```python
from build123d import *

# Parameters (mm, degrees)
SKETCH1_R           = 12.25
BOSS_EXTRUDE1_DEPTH = 280
CUT_EXTRUDE1_DEPTH  = 20


with BuildPart() as part:
    # Sketch1 → Boss-Extrude1 (new body)
    with BuildSketch(Plane.XY):
        Circle(SKETCH1_R)
    extrude(amount=BOSS_EXTRUDE1_DEPTH)

    # Sketch2 → Cut-Extrude1 (cut)
    with BuildSketch(Plane.XY.offset(280)):
        with BuildLine():
            Line((1, 6.75), (-1, 6.75))
            Line((-1, 6.75), (-1, 8.692669325))
            ThreePointArc((-1, 8.692669325), (-3.348480033, 8.083945909), (-5.439538645, 6.853752208))
            Line((-5.439538645, 6.853752208), (-4.065863992, 5.480077554))
            Line((-4.065863992, 5.480077554), (-5.480077554, 4.065863992))
            Line((-5.480077554, 4.065863992), (-6.853752208, 5.439538645))
            ThreePointArc((-6.853752208, 5.439538645), (-8.083945909, 3.348480033), (-8.692669325, 1))
            Line((-8.692669325, 1), (-6.75, 1))
            Line((-6.75, 1), (-6.75, -1))
            Line((-6.75, -1), (-8.692669325, -1))
            ThreePointArc((-8.692669325, -1), (-8.083945909, -3.348480033), (-6.853752208, -5.439538645))
            Line((-6.853752208, -5.439538645), (-5.480077554, -4.065863992))
            Line((-5.480077554, -4.065863992), (-4.065863992, -5.480077554))
            Line((-4.065863992, -5.480077554), (-5.439538645, -6.853752208))
            ThreePointArc((-5.439538645, -6.853752208), (-3.348480033, -8.083945909), (-1, -8.692669325))
            Line((-1, -8.692669325), (-1, -6.75))
            Line((-1, -6.75), (1, -6.75))
            Line((1, -6.75), (1, -8.692669325))
            ThreePointArc((1, -8.692669325), (3.348480033, -8.083945909), (5.439538645, -6.853752208))
            Line((5.439538645, -6.853752208), (4.065863992, -5.480077554))
            Line((4.065863992, -5.480077554), (5.480077554, -4.065863992))
            Line((5.480077554, -4.065863992), (6.853752208, -5.439538645))
            ThreePointArc((6.853752208, -5.439538645), (8.083945909, -3.348480033), (8.692669325, -1))
            Line((8.692669325, -1), (6.75, -1))
            Line((6.75, -1), (6.75, 1))
            Line((6.75, 1), (8.692669325, 1))
            ThreePointArc((8.692669325, 1), (8.083945909, 3.348480033), (6.853752208, 5.439538645))
            Line((6.853752208, 5.439538645), (5.480077554, 4.065863992))
            Line((5.480077554, 4.065863992), (4.065863992, 5.480077554))
            Line((4.065863992, 5.480077554), (5.439538645, 6.853752208))
            ThreePointArc((5.439538645, 6.853752208), (3.348480033, 8.083945909), (1, 8.692669325))
            Line((1, 8.692669325), (1, 6.75))
        make_face()
    extrude(amount=-CUT_EXTRUDE1_DEPTH, mode=Mode.SUBTRACT)


solid = part.part
```
Source: CAD feature listing. Evaluate the final solid. Frame: model axes, mm. Coordinates: 2 decimals unless noted, no trailing zeros. Loops run counter-clockwise (first coordinate to the right, second up) from the corner with the lowest first, then second, coordinate; pieces in that order, holes last. Notation, with made-up numbers: M -10,23.5 L -2,23.5 A11 ccw -2,42.5 Z; hole C 2.25,31 d4. An arc over 180 degrees is marked long. Use a Markdown table: item, result. Add a question column.
Q1. Material intervals for L1, parallel to Z at x = 8, y = 3; L2, parallel to Y at x = -10.25, z = 103; L3, parallel to Y at x = -2, z = 263.5, sorted ascending.
Q2. First-contact query: pin 1 (2 mm diameter, centred on x = -7.5, z = 273, fed in from +Y); pin 2 (0.6 mm diameter, centred on y = -7.5, z = 273, fed in from +X); pin 3 (10 mm diameter, centred on x = -9, y = 5, fed in from -Z); pin 4 (2 mm diameter, centred on y = 4.5, z = 63.5, fed in from -X). Flat tips, straight axial feed; report the tip coordinate or a pass-through.
Q3. Section query B-B, the plane z = 114. Return loops of the section in (x, y), and give its area (3 significant figures).
Q4. Draft query along Y for faces 1 (the cylindrical face through (-3.317, 8.097, 270.14)), 2 (the cylindrical face through (6.586, 10.329, 138.04)), 3 (the flat face through (5, -5, 280)). Return one class per face: pulls with the +Y half, pulls with the -Y half, needs draft (parallel to the pull), parting line crosses it, or undercut.
Result:
| question | item | result |
|---|---|---|
| 1 | L1 | z = 0 to 260 |
| 1 | L2 | y = -6.71 to 6.71 |
| 1 | L3 | y = -12.09 to -8.52, 8.52 to 12.09 |
| 2 | pin 1 | stops at y = 10.38 |
| 2 | pin 2 | stops at x = 9.91 |
| 2 | pin 3 | stops at z = 0 |
| 2 | pin 4 | stops at x = -11.74 |
| 3 | outline | C 0,0 d24.5 |
| 3 | area | 471 mm2 |
| 4 | face 1 | undercut |
| 4 | face 2 | parting line crosses it |
| 4 | face 3 | needs draft |
